from build123d import *

# Parameters (mm, degrees)
F1_DEPTH = 330.2


with BuildPart() as f1:
    # F0 (on Right) → F1 (new body)
    with BuildSketch(Plane.YZ):
        with BuildLine():
            Line((-28.115756, 44.895094), (-28.115756, -12.254906))
            Line((-28.115756, -12.254906), (-23.353256, -12.254906))
            Line((-23.353256, -12.254906), (-23.353256, 41.402594))
            ThreePointArc((-23.353256, 41.402594), (-21.865359, 44.994697), (-18.273256, 46.482594))
            Line((-18.273256, 46.482594), (35.384244, 46.482594))
            Line((35.384244, 46.482594), (35.384244, 51.245094))
            Line((35.384244, 51.245094), (-21.765756, 51.245094))
            ThreePointArc((-21.765756, 51.245094), (-26.255884, 49.385222), (-28.115756, 44.895094))
        make_face()
    extrude(amount=F1_DEPTH)


solid = f1.part
Could you check a few things on this model? Use its own coordinates, in mm. A direction names the side the tool comes from. Give positions to 0.01 mm unless a question says otherwise; leave off trailing zeros. Order: outer loops, then holes, each group sorted by start corner. A loop starts at its lowest first (then second) coordinate and runs counter-clockwise, first axis right, second up.
1. Suppose I cut it at C-C (y = 8.5). Write out the boundary of the cut face in (x, z), plus the area to 3 significant figures.
Answers below:
outline: (0, 46.48) - (330.2, 46.48) - (330.2, 51.25) - (0, 51.25) - close
area: 1,570 mm2
2. Suppose I cut it at A-A (x = 250.5). Write out the boundary of the cut face in (y, z).
Answers below:
outline: (-28.12, -12.25) - (-23.35, -12.25) - (-23.35, 41.4) arc R5.08 cw to (-18.27, 46.48) - (35.38, 46.48) - (35.38, 51.25) - (-21.77, 51.25) arc R6.35 ccw to (-28.12, 44.9) - close
3. Suppose I cut it at B-B (z = 18). Write out the boundary of the cut face in (x, y), plus the area to 3 significant figures.
Answers below:
outline: (0, -28.12) - (330.2, -28.12) - (330.2, -23.35) - (0, -23.35) - close
area: 1,570 mm2
4. I need wall thicknesses on L1, parallel to Z at x = 66.5, y = 22; L2, parallel to Y at x = 39.5, z = 32; L3, parallel to Z at x = 210.5, y = -24. Which ranges of each line are inside material? Lowest first, please.
Answers below:
L1: z = 46.48 to 51.25
L2: y = -28.12 to -23.35
L3: z = -12.25 to 50.84
5. For pin 1 (12 mm diameter, centred on x = 161.5, y = 12, fed in from -Z); pin 2 (1.5 mm diameter, centred on x = 142.5, z = 19.5, fed in from +Y), each with a flat end and sliding along its axis, tell me the tip position at first contact or that it passes through.
Answers below:
pin 1: stops at z = 46.48
pin 2: stops at y = -23.35
6. Which directions (+Z, -Z, +X, -X, +Y, -Y) give clear straight access to the entire face, cutting with the end or side of a thin tool? Please do faces 1 (the flat face through (163, 7, 51.245)), 2 (the flat face through (163, -23.353, 14)).
Answers below:
face 1: +Z, +X, -X, +Y, -Y
face 2: -Z, +X, -X, +Y
